```python
from build123d import *
from build123d.topology import SkipClean

# Parameters (mm, degrees)
EXTRUDE_1_DEPTH     = 2
EXTRUDE_2_DEPTH     = 17
EXTRUDE_3_DEPTH     = 5
HOLE_WIZARD_M31_D   = 3.4
EXTRUDE_4_DEPTH     = 11
CUT_EXTRUDE_1_DEPTH = 11
HOLE_WIZARD_M31_2_D = 2.5


with BuildPart() as part:
    # Sketch 1 → Extrude 1 (new body)
    with BuildSketch(Plane(origin=(0, 0, 0), x_dir=(1, 0, 0), z_dir=(0, 1, 0))):
        with BuildLine():
            Line((22.325097984, -2.8), (25.3, -2.8))
            ThreePointArc((25.3, -2.8), (28.1, 0), (25.3, 2.8))
            Line((25.3, 2.8), (22.325097984, 2.8))
            ThreePointArc((22.325097984, 2.8), (15.909902577, 15.909902577), (2.8, 22.325097984))
            Line((2.8, 22.325097984), (2.8, 25.3))
            ThreePointArc((2.8, 25.3), (0, 28.1), (-2.8, 25.3))
            Line((-2.8, 25.3), (-2.8, 22.325097984))
            ThreePointArc((-2.8, 22.325097984), (-15.909902577, 15.909902577), (-22.325097984, 2.8))
            Line((-22.325097984, 2.8), (-25.3, 2.8))
            ThreePointArc((-25.3, 2.8), (-28.1, 0), (-25.3, -2.8))
            Line((-25.3, -2.8), (-22.325097984, -2.8))
            ThreePointArc((-22.325097984, -2.8), (-15.909902577, -15.909902577), (-2.8, -22.325097984))
            Line((-2.8, -22.325097984), (-2.8, -25.3))
            ThreePointArc((-2.8, -25.3), (0, -28.1), (2.8, -25.3))
            Line((2.8, -25.3), (2.8, -22.325097984))
            ThreePointArc((2.8, -22.325097984), (14.4243682, -14.4243682), (22.325097984, -2.8))
        make_face()
        with BuildLine():
            ThreePointArc((18.417505142, -1.745137346), (-13.081475452, 13.081475452), (1.745137346, -18.417505142))
            ThreePointArc((1.745137346, -18.417505142), (11.595941075, -11.595941075), (18.417505142, -1.745137346))
        make_face(mode=Mode.SUBTRACT)
    extrude(amount=EXTRUDE_1_DEPTH)

    # Sketch 2 → Extrude 2 (add)
    with BuildSketch(Plane(origin=(0, 2, 0), x_dir=(1, 0, 0), z_dir=(0, 1, 0))):
        with BuildLine():
            Line((20.003268693, 4.485447761), (23.557492243, -11.364940531))
            ThreePointArc((23.557492243, -11.364940531), (14.4243682, -14.4243682), (11.364940531, -23.557492243))
            Line((11.364940531, -23.557492243), (-4.485447761, -20.003268693))
            ThreePointArc((-4.485447761, -20.003268693), (-14.495689014, -14.495689014), (-20.003268693, -4.485447761))
            Line((-20.003268693, -4.485447761), (-24.05725546, 13.593680769))
            ThreePointArc((-24.05725546, 13.593680769), (-15.909902577, 15.909902577), (-13.593680769, 24.05725546))
            Line((-13.593680769, 24.05725546), (4.485447761, 20.003268693))
            ThreePointArc((4.485447761, 20.003268693), (14.495689014, 14.495689014), (20.003268693, 4.485447761))
        make_face()
        with BuildLine():
            ThreePointArc((1.745137346, -18.417505142), (11.595941075, -11.595941075), (18.417505142, -1.745137346))
            ThreePointArc((18.417505142, -1.745137346), (-13.081475452, 13.081475452), (1.745137346, -18.417505142))
        make_face(mode=Mode.SUBTRACT)
    extrude(amount=EXTRUDE_2_DEPTH)

    # Sketch 3 → Extrude 3 (add)
    with BuildSketch(Plane(origin=(0, 19, 0), x_dir=(1, 0, 0), z_dir=(0, 1, 0))):
        with BuildLine():
            Line((20.003268693, 4.485447761), (25.76965455, -21.23028272))
            ThreePointArc((25.76965455, -21.23028272), (24.748737342, -24.748737342), (21.23028272, -25.76965455))
            Line((21.23028272, -25.76965455), (-4.485447761, -20.003268693))
            ThreePointArc((-4.485447761, -20.003268693), (-14.495689014, -14.495689014), (-20.003268693, -4.485447761))
            Line((-20.003268693, -4.485447761), (-25.76965455, 21.23028272))
            ThreePointArc((-25.76965455, 21.23028272), (-24.748737342, 24.748737342), (-21.23028272, 25.76965455))
            Line((-21.23028272, 25.76965455), (4.485447761, 20.003268693))
            ThreePointArc((4.485447761, 20.003268693), (14.495689014, 14.495689014), (20.003268693, 4.485447761))
        make_face()
    extrude(amount=EXTRUDE_3_DEPTH)

    # Hole Wizard M31 (through all)
    with Locations(Plane(origin=(0, 0, 0), x_dir=(-1, 0, 0), z_dir=(0, -1, 0))):
        with Locations((-22.061731573, -22.061731573), (22.061731573, 22.061731573)):
            Hole(HOLE_WIZARD_M31_D / 2)

    # Sketch 6 → Extrude 4 (add)
    with SkipClean():  # the faces are left unmerged after this step: merging them gives an invalid solid
        with BuildSketch(Plane(origin=(0, 2, 0), x_dir=(1, 0, 0), z_dir=(0, 1, 0))):
            with BuildLine():
                Line((0.75, 20.840889586), (-0.75, 21.177243196))
                Line((-0.75, 21.177243196), (-0.75, 22.602315808))
                ThreePointArc((-0.75, 22.602315808), (0, 28.1), (0.75, 22.602315808))
                Line((0.75, 22.602315808), (0.75, 20.840889586))
            make_face()
            with BuildLine():
                Line((-21.177243196, 0.75), (-22.602315808, 0.75))
                ThreePointArc((-22.602315808, 0.75), (-28.1, 0), (-22.602315808, -0.75))
                Line((-22.602315808, -0.75), (-20.840889586, -0.75))
                Line((-20.840889586, -0.75), (-21.177243196, 0.75))
            make_face()
            with BuildLine():
                Line((21.177243196, -0.75), (20.840889586, 0.75))
                Line((20.840889586, 0.75), (22.602315808, 0.75))
                ThreePointArc((22.602315808, 0.75), (28.1, 0), (22.602315808, -0.75))
                Line((22.602315808, -0.75), (21.177243196, -0.75))
            make_face()
            with BuildLine():
                Line((-0.75, -20.840889586), (0.75, -21.177243196))
                Line((0.75, -21.177243196), (0.75, -22.602315808))
                ThreePointArc((0.75, -22.602315808), (0, -28.1), (-0.75, -22.602315808))
                Line((-0.75, -22.602315808), (-0.75, -20.840889586))
            make_face()
        extrude(amount=EXTRUDE_4_DEPTH)

    # Sketch 7 → Cut-Extrude 1 (cut)
    with SkipClean():  # the faces are left unmerged after this step: merging them gives an invalid solid
        with BuildSketch(Plane.XZ.offset(-19)):
            with BuildLine():
                ThreePointArc((18.417505142, 1.745137346), (11.595941075, 11.595941075), (1.745137346, 18.417505142))
                ThreePointArc((1.745137346, 18.417505142), (-13.081475452, -13.081475452), (18.417505142, 1.745137346))
            make_face()
        extrude(amount=-CUT_EXTRUDE_1_DEPTH, mode=Mode.SUBTRACT)

    # Hole Wizard M31 2 (through all)
    with Locations(Plane(origin=(0, 0, 0), x_dir=(-1, 0, 0), z_dir=(0, -1, 0))):
        with Locations((0, -25.3), (-25.3, 0), (0, 25.3), (25.3, 0)):
            Hole(HOLE_WIZARD_M31_2_D / 2)


solid = part.part
```
Read the model definition and answer for the solid it produces. Units are mm, in the model's axes. A direction names the side the tool comes from. Give positions to 0.01 mm unless a question says otherwise; leave off trailing zeros. Order: outer loops, then holes, each group sorted by start corner. A loop starts at its lowest first (then second) coordinate and runs counter-clockwise, first axis right, second up.
(1) Find section B-B (y = 10.75). Give the number of separate pieces and of enclosed holes in the cut face, plus the area to 3 significant figures.
(2) For faces 1 (the flat face through (0, 13, 23.6)), 2 (the flat face through (2.8, 1, -24)), 3 (the flat face through (-2, 2, -22)), determine the directions among +Z, -Z, +X, -X, +Y, -Y from which every point of the face is accessible in a straight line to the end or side of a thin tool.
(3) Find section C-C (z = 7.5). Give the vertices of the cut face in (x, y), plus the area to 3 significant figures.
(4) Given pin 1 (1 mm diameter, centred on y = 14.5, z = -1, fed in from +X); pin 2 (12 mm diameter, centred on y = 14, z = 13.5, fed in from +X); pin 3 (1 mm diameter, centred on y = 0.5, z = 23.5, fed in from +X), each flat-ended and moving along its own axis, determine where each tip first touches the part or whether it passes through.
(5) Find section D-D (x = -5.5). Give the vertices of the cut face in (y, z), plus the area to 3 significant figures.
(6) Find section A-A (y = 18.25). Give the vertices of the cut face in (x, z).
(7) Straight lines are drawn through the part: L1, parallel to Z at x = 0, y = 6.75; L2, parallel to Z at x = 7.5, y = 10; L3, parallel to X at y = 17, z = 0.5. For each, find the intervals that lie inside material, in ascending order.
Result sheet:
1. separate pieces: 1
1. enclosed holes: 5
1. area: 550 mm2
2. face 1: +Z, -X, +Y
2. face 2: -Z, +X, +Y, -Y
2. face 3: +Y
3. outline: (-21.21, 0) - (-16.91, 0) - (-16.91, 24) - (-19.08, 24) - (-19.08, 2) - (-21.21, 2) - close; (15.08, 0) - (19.88, 0) - (19.88, 2) - (22.69, 2) - (22.69, 24) - (15.08, 24) - close
3. area: 233 mm2
4. pin 1: stops at x = 20.9
4. pin 2: stops at x = 24.78
4. pin 3: stops at x = 2.8
5. outline: (0, -21.82) - (2, -21.82) - (2, -22.24) - (24, -22.24) - (24, -17.66) - (0, -17.66) - close; (0, 17.66) - (24, 17.66) - (24, 19.75) - (2, 19.75) - (2, 21.82) - (0, 21.82) - close
5. area: 163 mm2
6. outline: (-24.06, -13.59) arc R8.7 cw to (-13.59, -24.06) - (4.49, -20) arc R20.5 ccw to (20, -4.49) - (23.56, 11.36) arc R10.8 cw to (11.36, 23.56) - (-4.49, 20) arc R20.5 ccw to (-20, 4.49) - close; hole (1.75, 18.42) arc R18.5 ccw (long way) to (18.42, 1.75) arc R33.51 ccw to start
7. L1: z = -28.1 to -26.55, -24.05 to -18.5, 18.5 to 24.05, 26.55 to 28.1
7. L2: z = -19.08 to -16.91, 15.08 to 22.69
7. L3: x = -20.9 to -18.49, 18.49 to 21.12
